Geometry check sheet. Reference: drawing and pictorial views, mm from the part's lowest x, y, z. Coordinates: 2 decimals unless noted, no trailing zeros. Loops run counter-clockwise (first coordinate to the right, second up) from the corner with the lowest first, then second, coordinate; pieces in that order, holes last.
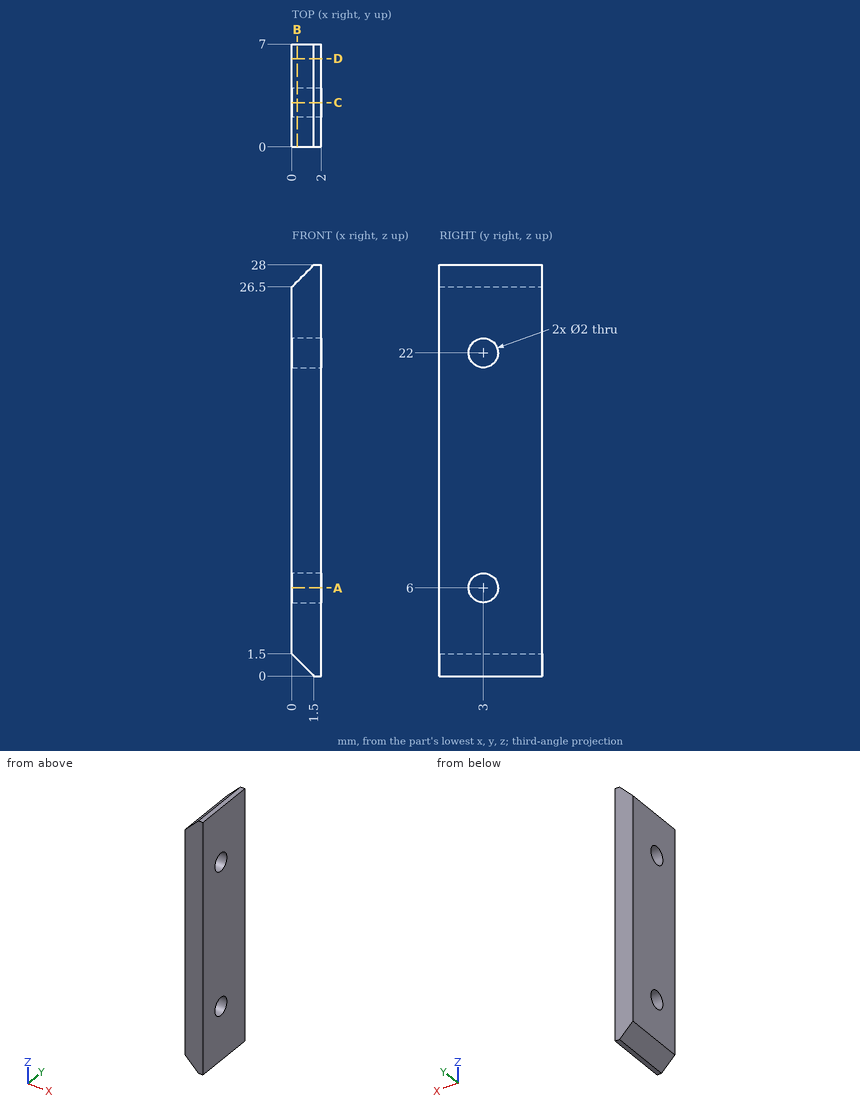
1) Section check B-B on x = 0.35. Record the cut outline in (y, z).
Data:
outline: (0, 1.15) - (7, 1.15) - (7, 26.85) - (0, 26.85) - close; hole circle Ø2 at (3, 6); hole circle Ø2 at (3, 22)
2) Section check D-D on y = 6. Record the cut outline in (x, z), and give its area (4 significant figures).
Data:
outline: (0, 1.5) - (1.5, 0) - (2, 0) - (2, 28) - (1.5, 28) - (0, 26.5) - close
area: 53.75 mm2
3) Material ranges on probe 1 along Y at (x, z) = (1.35, 22); probe 2 along Z at (x, y) = (1.3, 3); probe 3 along Z at (x, y) = (1.45, 3), recorded low to high.
Data:
probe 1: y = 0 to 2, 4 to 7
probe 2: z = 0.2 to 5, 7 to 21, 23 to 27.8
probe 3: z = 0.05 to 5, 7 to 21, 23 to 27.95
4) Section check A-A on z = 6. Record the cut outline in (x, y).
Data:
outline: (0, 0) - (2, 0) - (2, 2) - (0, 2) - close; (0, 4) - (2, 4) - (2, 7) - (0, 7) - close
5) Depth check by flat-ended pin: pin 1 (1.8 mm diameter, centred on y = 3, z = 22, fed in from +X); pin 2 (1 mm diameter, centred on x = 1.5, z = 7.5, fed in from -Y). Enter the tip coordinate at first touch or a pass-through.
Data:
pin 1: passes through
pin 2: stops at y = 0
6) Section check C-C on y = 3. Record the cut outline in (x, z).
Data:
outline: (0, 1.5) - (1.5, 0) - (2, 0) - (2, 5) - (0, 5) - close; (0, 7) - (2, 7) - (2, 21) - (0, 21) - close; (0, 23) - (2, 23) - (2, 28) - (1.5, 28) - (0, 26.5) - close
